Source: CAD feature listing. Evaluate the final solid. Frame: model axes, mm. A direction names the side the tool comes from. Coordinates: 2 decimals unless noted, no trailing zeros. Write each loop counter-clockwise with the first axis right and the second up, starting at its lowest first coordinate (ties: lowest second). Pieces come first, ordered by that corner, then holes. Notation, with made-up numbers: (4, 57.25) -> (50, 57.25) arc R24 ccw to (50, 92.25) -> close; hole circle Ø3 at (63.25, 60). An arc over 180 degrees is marked (long way). Write item = value, one per line.
from build123d import *

# Parameters (mm, degrees)
F1_DEPTH = 14
F2_R     = 3
F3_DEPTH = 38.001
F4_SIZE  = 1
F5_R     = 2
F6_DEPTH = 42.001
F7_ANGLE = 90


with BuildPart() as f1:
    # F0 (on Top) → F1 (new body)
    with BuildSketch(Plane.XY):
        with BuildLine():
            Line((-21, 6), (-21, 0))
            Line((-21, 0), (21, 0))
            Line((21, 0), (21, 6))
            Line((21, 6), (11, 6))
            Line((11, 6), (8, 38))
            Line((8, 38), (1, 38))
            Line((1, 38), (1, 28.91608))
            ThreePointArc((1, 28.91608), (4.582576, 26.872983), (6, 23))
            ThreePointArc((6, 23), (-3.872983, 18.417424), (-1, 28.91608))
            Line((-1, 28.91608), (-1, 38))
            Line((-1, 38), (-8, 38))
            Line((-8, 38), (-11, 6))
            Line((-11, 6), (-21, 6))
        make_face()
    extrude(amount=F1_DEPTH)

    # F2 (on face) → F3 (cut, through all)
    with BuildSketch(Plane.XZ):
        with Locations((-16, 7)):
            Circle(F2_R)
        with Locations((16, 7)):
            Circle(F2_R)
    extrude(amount=-F3_DEPTH, mode=Mode.SUBTRACT)

    # F4
    f4_edges = [f1.edges().sort_by_distance(p)[0] for p in [
        (0, 17, 14),
        (0, 17, 0),
    ]]
    chamfer(f4_edges, length=F4_SIZE)

    # F5 (on face) → F6 (cut, through all)
    with BuildSketch(Plane(origin=(-21, 0, 0), x_dir=(0, -1, 0), z_dir=(-1, 0, 0))):
        with Locations((-34, 7)):
            Circle(F5_R)
    extrude(amount=-F6_DEPTH, mode=Mode.SUBTRACT)


with BuildPart() as f1_1:
    # F7: moved
    add(f1.part.rotate(Axis((0, 0, 0), (1, 0, 0)), F7_ANGLE))


solid = f1_1.part
1) First-contact query: pin 1 Ø5 at (y, z) = (-5.5, 16) entering from -X; pin 2 Ø2.5 at (y, z) = (-4, 34.5) entering from +X; pin 3 Ø8 at (x, y) = (-16, -7) entering from -Z; pin 4 Ø8 at (x, y) = (16, -7) entering from +Z. Flat tips, straight axial feed; report the tip coordinate or a pass-through.
Answer block:
pin_1 = -10.3
pin_2 = 8.45
pin_3 = 0
pin_4 = 6
2) Reachability of faces 5 (the cylindrical face through (13.6, -5.2, 3)), 6 (the flat face through (1, -5, 33)), 7 (the flat face through (-15.9, -3.8, 6)), 8 (the flat face through (16.1, -3.8, 6)), 9 (the flat face through (5, -7, 38)) from +Z, -Z, +X, -X, +Y, -Y: full face, straight path, thin tool, end or side. Return the list, or none.
Answer block:
face_5 = +Z, -Z
face_6 = +Z, +Y, -Y
face_7 = +Z, -X, +Y, -Y
face_8 = +Z, +X, +Y, -Y
face_9 = +Z, +X, -X, +Y, -Y
3) Material intervals for probe 1 along X at (y, z) = (-7, 4.4); probe 2 along Y at (x, z) = (16, 1.6); probe 3 along Z at (x, y) = (2, -5.75), sorted ascending. Write a range as [from, to].
Answer block:
probe_1 = [-21, -19], [-13, 13], [19, 21]
probe_2 = [-14, -10], [-4, 0]
probe_3 = [0, 17.34], [28.66, 32.44], [35.56, 38]
4) Cut plane C-C, the plane z = 4. Output: boundary loops of the cut face in (x, y), and give its area (3 significant figures).
Answer block:
outline = (-21, -14) -> (21, -14) -> (21, 0) -> (-21, 0) -> close; hole circle Ø6 at (-16, -7); hole circle Ø6 at (16, -7)
area = 531 mm2
5) Pull-direction query (Y, two-part tool) for faces 1 (the cylindrical face through (-19, -7, 3)), 2 (the flat face through (0, -14, 11)), 3 (the flat face through (-21, -7, 3)), 4 (the flat face through (0, 0, 11)); classes: +Y half, -Y half, draft (parallel to the pull), parting line (faces both ways), or undercut.
Answer block:
face_1 = undercut
face_2 = -Y half
face_3 = draft
face_4 = +Y half
6) Cut plane A-A, the plane x = -16. Output: boundary loops of the cut face in (y, z), and give its area (3 significant figures).
Answer block:
outline = (-14, 0) -> (-10, 0) -> (-10, 6) -> (-14, 6) -> close; (-4, 0) -> (0, 0) -> (0, 6) -> (-4, 6) -> close
area = 48.0 mm2
7) Cut plane B-B, the plane y = -7. Output: boundary loops of the cut face in (x, z), and give its area (3 significant figures).
Answer block:
outline = (-21, 0) -> (-19, 0) -> (-19, 6) -> (-21, 6) -> close; (-13, 0) -> (13, 0) -> (13, 6) -> (11, 6) -> (8.56, 32) -> (1, 32) -> (1, 28.92) arc R6 cw (long way) to (-1, 28.92) -> (-1, 32) -> (-8.56, 32) -> (-11, 6) -> (-13, 6) -> close; (-8.19, 36) -> (-1, 36) -> (-1, 38) -> (-8, 38) -> close; (1, 36) -> (8.19, 36) -> (8, 38) -> (1, 38) -> close; (19, 0) -> (21, 0) -> (21, 6) -> (19, 6) -> close
area = 598 mm2
8) Cut plane D-D, the plane y = -10.75. Output: boundary loops of the cut face in (x, z).
Answer block:
outline = (-21, 0) -> (21, 0) -> (21, 6) -> (11, 6) -> (8, 38) -> (1, 38) -> (1, 28.92) arc R6 cw (long way) to (-1, 28.92) -> (-1, 38) -> (-8, 38) -> (-11, 6) -> (-21, 6) -> close
